Model file for the job. Use its own axes, mm. Face numbers are marked on the shaded views. Coordinates: 2 decimals unless noted, no trailing zeros. Write each loop counter-clockwise with the first axis right and the second up, starting at its lowest first coordinate (ties: lowest second). Pieces come first, ordered by that corner, then holes.
Q1. Band-saw the part on C-C, the plane y = -0.9. Write the cut outline in (x, z).
Q2. Pull direction Z, two halves, no side cores. Call the marked faces 1, 2 and 3: released by +Z, released by -Z, zero draft, split by the parting line, or undercut.
Q3. Drill centre lines: probe 1 along Z at (x, y) = (0, -3.3); probe 2 along Z at (x, y) = (-0.5, -0.85); probe 3 along Z at (x, y) = (-9, -1.15). Where is each one in solid material? Low to high.
Q4. Band-saw the part on B-B, the plane x = 0. Write the cut outline in (y, z) (1 decimal), plus the area to 3 significant figures.
Q5. Band-saw the part on D-D, the plane y = -2.65. Write the cut outline in (x, z) (1 decimal), plus the area to 3 significant figures.
Q6. Pin check, flat tips, straight feed: P1, Ø1.5, axis at x = 0, z = 12.446, coming from the +Y side; P2, Ø1, axis at x = 3.5, y = -3.5, coming from the +Z side. Stop position of each tip, or through.
Q7. Band-saw the part on A-A, the plane z = 0. Write the cut outline in (x, y) (3 decimals).
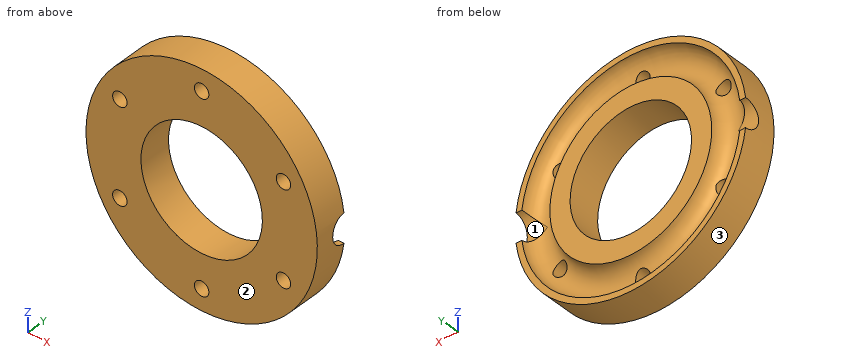
from build123d import *
from build123d.topology import SkipClean

# Parameters (mm, degrees)
SKETCH1_R                     = 10.414
SKETCH1_R_2                   = 8.001
BOSS_EXTRUDE1_DEPTH           = 4.318
BOSS_EXTRUDE2_START           = 4.318
SKETCH2_R                     = 15.24
SKETCH2_R_2                   = 8.001
BOSS_EXTRUDE2_DEPTH           = 4.318
SKETCH3_R                     = 1.905
CUT_EXTRUDE1_REACH            = 23.981
SKETCH4_R                     = 0.9525
CIRPATTERN1_COUNT             = 6
CUT_EXTRUDE2_START            = -4.318
SKETCH5_R                     = 10.414
CUT_EXTRUDE2_DEPTH            = 4.318
CUT_EXTRUDE3_REACH            = 36.35
CUT_EXTRUDE3_END_MAJOR_RADIUS = 12.573
CUT_EXTRUDE3_END_MINOR_RADIUS = 1.905
SKETCH8_R                     = 1.905
CIRPATTERN2_COUNT             = 2


with BuildPart() as part:
    # Sketch1 → Boss-Extrude1 (new body)
    with BuildSketch(Plane(origin=(0, 0, 0), x_dir=(1, 0, 0), z_dir=(0, 1, 0))):
        with Locations(Location((0, 0, 0), (0, 0, 270))):
            Circle(SKETCH1_R)
        with Locations(Location((0, 0, 0), (0, 0, 270))):
            Circle(SKETCH1_R_2, mode=Mode.SUBTRACT)
    extrude(amount=BOSS_EXTRUDE1_DEPTH)

    # Sketch2 → Boss-Extrude2 (add)
    with SkipClean():  # the faces are left unmerged after this step: merging them gives an invalid solid
        with BuildSketch(Plane.XZ.offset(BOSS_EXTRUDE2_START)):
            with Locations(Location((0, 0, 0), (0, 0, 270))):
                Circle(SKETCH2_R)
            with Locations(Location((0, 0, 0), (0, 0, 270))):
                Circle(SKETCH2_R_2, mode=Mode.SUBTRACT)
        extrude(amount=-BOSS_EXTRUDE2_DEPTH)

    # Sketch3 → Cut-Revolve1 (revolve, cut)
    with SkipClean():  # the faces are left unmerged after this step: merging them gives an invalid solid
        with BuildSketch(Plane.XY, mode=Mode.PRIVATE) as cut_revolve1_sk:
            with Locations((12.573, 0)):
                Circle(SKETCH3_R)
        revolve(cut_revolve1_sk.sketch.rotate(Axis((0, 55, 0), (0, -1, 0)), 270), axis=Axis((0, 55, 0), (0, -1, 0)), mode=Mode.SUBTRACT)

    # Sketch4 → Cut-Extrude1 (cut, up to next)
    with BuildSketch(Plane(origin=(0, 0, 0), x_dir=(1, 0, 0), z_dir=(0, 1, 0)), mode=Mode.PRIVATE) as cut_extrude1_sk1:
        with Locations(Location((0, 12.446, 0), (0, 0, 132.863672282))):
            Circle(SKETCH4_R)
    cut_extrude1_tool1 = extrude(cut_extrude1_sk1.sketch, amount=-CUT_EXTRUDE1_REACH, mode=Mode.PRIVATE) & part.part
    cut_extrude1 = cut_extrude1_tool1.solids().sort_by_distance((0, 0, -12.446))[0]
    add(cut_extrude1, mode=Mode.SUBTRACT)

    # CirPattern1: Cut-Extrude1 ×6 about axis
    with SkipClean():  # the faces are left unmerged after this step: merging them gives an invalid solid
        cirpattern1_axis = Axis((0, 0, 0), (0, 1, 0))
        for i in range(1, CIRPATTERN1_COUNT):
            add(cut_extrude1.rotate(cirpattern1_axis, i * 360 / CIRPATTERN1_COUNT), mode=Mode.SUBTRACT)

    # Sketch5 → Cut-Extrude2 (cut)
    with BuildSketch(Plane(origin=(0, 4.318, 0), x_dir=(1, 0, 0), z_dir=(0, 1, 0)).offset(CUT_EXTRUDE2_START)):
        Circle(SKETCH5_R)
    extrude(amount=CUT_EXTRUDE2_DEPTH, mode=Mode.SUBTRACT)

    # Cut-Extrude3: up to this torus (the profile starts outside it)
    cut_extrude3_end = Plane(origin=(0, 0, 0), z_dir=(0, 1, 0)) * Torus(CUT_EXTRUDE3_END_MAJOR_RADIUS, CUT_EXTRUDE3_END_MINOR_RADIUS, mode=Mode.PRIVATE)
    # Sketch8 → Cut-Extrude3 (cut, up to the surface)
    with BuildSketch(Plane(origin=(15.24, 0, 0), x_dir=(0, 0, -1), z_dir=(1, 0, 0)), mode=Mode.PRIVATE) as cut_extrude3_sk1:
        Circle(SKETCH8_R)
    cut_extrude3_tool1 = extrude(cut_extrude3_sk1.sketch, amount=-CUT_EXTRUDE3_REACH, mode=Mode.PRIVATE) - cut_extrude3_end
    cut_extrude3 = cut_extrude3_tool1.solids().sort_by_distance((15.24, 0, 0))[0]
    add(cut_extrude3, mode=Mode.SUBTRACT)

    # CirPattern2: Cut-Extrude3 ×2 about axis
    cirpattern2_axis = Axis((0, 55, 0), (0, -1, 0))
    for i in range(1, CIRPATTERN2_COUNT):
        add(cut_extrude3.rotate(cirpattern2_axis, i * 360 / CIRPATTERN2_COUNT), mode=Mode.SUBTRACT)


solid = part.part
Answer sheet:
1. outline: (-15.15, -1.68) arc R15.24 ccw to (15.15, -1.68) - (14.15, -1.68) arc R14.25 cw to (-14.15, -1.68) - close; (-15.15, 1.68) - (-14.15, 1.68) arc R14.25 cw to (14.15, 1.68) - (15.15, 1.68) arc R15.24 ccw to start; circle Ø21.79 at (0, 0); hole circle Ø16 at (0, 0)
2. face 1: undercut
2. face 2: zero draft
2. face 3: split by the parting line
3. probe 1: z = -15.24 to -13.4, -11.49 to -8, 8 to 11.49, 13.4 to 15.24
3. probe 2: z = -15.23 to -14.27, -10.86 to -7.99, 7.99 to 10.86, 14.27 to 15.23
3. probe 3: z = -12.3 to -10.84, -6.42 to 6.42, 10.84 to 12.3
4. outline: (-4.3, -15.2) - (0, -15.2) - (0, -14.5) arc R1.9 cw to (-1.7, -13.4) - (-4.3, -13.4) - close; (-4.3, -11.5) - (-1.6, -11.5) arc R1.9 cw to (0, -10.7) - (0, -8) - (-4.3, -8) - close; (-4.3, 8) - (0, 8) - (0, 10.7) arc R1.9 cw to (-1.6, 11.5) - (-4.3, 11.5) - close; (-4.3, 13.4) - (-1.7, 13.4) arc R1.9 cw to (0, 14.5) - (0, 15.2) - (-4.3, 15.2) - close
4. area: 41.6 mm2
5. outline: circle Ø30.5 at (0, 0); hole circle Ø1.9 at (-10.8, -6.2); hole circle Ø1.9 at (-10.8, 6.2); hole circle Ø16 at (0, 0); hole circle Ø1.9 at (0, -12.4); hole circle Ø1.9 at (0, 12.4); hole circle Ø1.9 at (10.8, -6.2); hole circle Ø1.9 at (10.8, 6.2)
5. area: 511 mm2
6. P1: passes through
6. P2: stops at z = 14.94
7. outline: (-15.24, -4.318) - (-8.001, -4.318) - (-8.001, 0) - (-10.668, 0) arc R1.905 cw to (-12.573, -1.905) - (-15.24, -1.905) - close; (8.001, -4.318) - (15.24, -4.318) - (15.24, -1.905) - (12.573, -1.905) arc R1.905 cw to (10.668, 0) - (8.001, 0) - close
